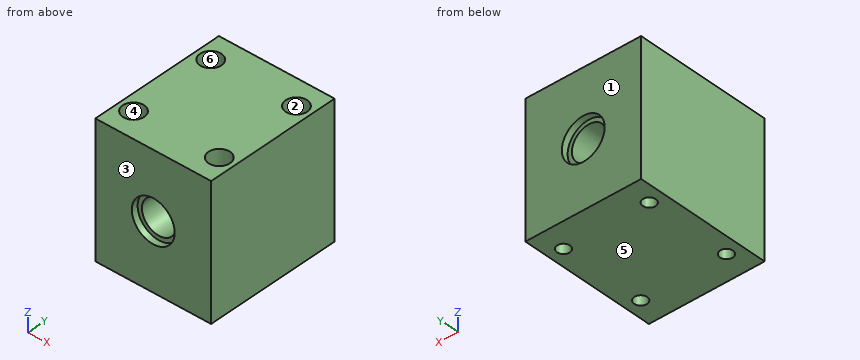
from build123d import *

# Parameters (mm, degrees)
SCHIZZO1_W                   = 27
SCHIZZO1_H                   = 32
ESTRUSIONE_ESTRUSIONE1_DEPTH = 31
SCHIZZO2_R                   = 1.5
TAGLIO_ESTRUSIONE1_DEPTH     = 32
SCHIZZO3_R                   = 4
TAGLIO_ESTRUSIONE2_DEPTH     = 33
SCHIZZO4_R                   = 5
TAGLIO_ESTRUSIONE5_DEPTH     = 1.5
SCHIZZO5_R                   = 5
TAGLIO_ESTRUSIONE6_DEPTH     = 1.5
SCHIZZO6_R                   = 2.5
TAGLIO_ESTRUSIONE7_DEPTH     = 15


with BuildPart() as part:
    # Schizzo1 → Estrusione-Estrusione1 (new body)
    with BuildSketch(Plane.XY):
        Rectangle(SCHIZZO1_W, SCHIZZO1_H)
    extrude(amount=ESTRUSIONE_ESTRUSIONE1_DEPTH)

    # Schizzo2 → Taglio-Estrusione1 (cut, through all)
    with BuildSketch(Plane(origin=(0, 0, 0), x_dir=(-1, 0, 0), z_dir=(0, 0, -1))):
        with Locations((-10, 10)):
            Circle(SCHIZZO2_R)
        with Locations((10, 10)):
            Circle(SCHIZZO2_R)
        with Locations((10, -10)):
            Circle(SCHIZZO2_R)
        with Locations((-10, -10)):
            Circle(SCHIZZO2_R)
    extrude(amount=-TAGLIO_ESTRUSIONE1_DEPTH, mode=Mode.SUBTRACT)

    # Schizzo3 → Taglio-Estrusione2 (cut, through all)
    with BuildSketch(Plane(origin=(0, 16, 0), x_dir=(1, 0, 0), z_dir=(0, 1, 0))):
        with Locations((0, -15.5)):
            Circle(SCHIZZO3_R)
    extrude(amount=-TAGLIO_ESTRUSIONE2_DEPTH, mode=Mode.SUBTRACT)

    # Schizzo4 → Taglio-Estrusione5 (cut)
    with BuildSketch(Plane(origin=(0, 16, 0), x_dir=(1, 0, 0), z_dir=(0, 1, 0))):
        with Locations((0, -15.5)):
            Circle(SCHIZZO4_R)
    extrude(amount=-TAGLIO_ESTRUSIONE5_DEPTH, mode=Mode.SUBTRACT)

    # Schizzo5 → Taglio-Estrusione6 (cut)
    with BuildSketch(Plane.XZ.offset(16)):
        with Locations((0, 15.5)):
            Circle(SCHIZZO5_R)
    extrude(amount=-TAGLIO_ESTRUSIONE6_DEPTH, mode=Mode.SUBTRACT)

    # Schizzo6 → Taglio-Estrusione7 (cut)
    with BuildSketch(Plane.XY.offset(31)):
        with Locations((-10, 10)):
            Circle(SCHIZZO6_R)
        with Locations((10, 10)):
            Circle(SCHIZZO6_R)
        with Locations((10, -10)):
            Circle(SCHIZZO6_R)
        with Locations((-10, -10)):
            Circle(SCHIZZO6_R)
    extrude(amount=-TAGLIO_ESTRUSIONE7_DEPTH, mode=Mode.SUBTRACT)


solid = part.part
Build history of the part. All positions in model axes, mm. Face numbers are marked on the shaded views. A direction names the side the tool comes from. Give positions to 0.01 mm unless a question says otherwise; leave off trailing zeros. Order: outer loops, then holes, each group sorted by start corner. A loop starts at its lowest first (then second) coordinate and runs counter-clockwise, first axis right, second up. Notation, with made-up numbers: M 18,15.25 L 55,15.25 A36 ccw 55,52.25 Z; hole C 50.5,49 d11. An arc over 180 degrees is marked long. Put each result on its own line as item: value.
Item 1: Slice it at B-B, the plane y = 10. Write the cut outline in (x, z).
From the geometry:
outline: M -13.5,0 L -11.5,0 L -11.5,16 L -12.5,16 L -12.5,31 L -13.5,31 Z; M -8.5,0 L 8.5,0 L 8.5,16 L 7.5,16 L 7.5,31 L -7.5,31 L -7.5,16 L -8.5,16 Z; M 11.5,0 L 13.5,0 L 13.5,31 L 12.5,31 L 12.5,16 L 11.5,16 Z; hole C 0,15.5 d8
Item 2: Slice it at D-D, the plane z = 27.5. Write the cut outline in (x, y), plus the area to 3 significant figures.
From the geometry:
outline: M -13.5,-16 L 13.5,-16 L 13.5,16 L -13.5,16 Z; hole C -10,-10 d5; hole C -10,10 d5; hole C 10,-10 d5; hole C 10,10 d5
area: 785 mm2
Item 3: Probe line 1 (Y direction, x = -10, z = 8); line 2 (Y direction, x = -10, z = 23.75); line 3 (X direction, y = -7.5, z = 15.5). List the from-to ranges inside material, lowest first. Write a range as [from, to].
From the geometry:
line 1: y = [-16, -11.5], [-8.5, 8.5], [11.5, 16]
line 2: y = [-16, -12.5], [-7.5, 7.5], [12.5, 16]
line 3: x = [-13.5, -4], [4, 13.5]
Item 4: Flat gauge pins, fed straight in: pin 1 Ø1.5 at (x, y) = (-9.5, -10.5) entering from +Z; pin 2 Ø1.5 at (x, y) = (10, 9) entering from +Z; pin 3 Ø4.5 at (x, y) = (-10, -10) entering from -Z; pin 4 Ø5 at (x, z) = (2, 15.5) entering from -Y. Where does each tip first touch, or does it go through?
From the geometry:
pin 1: passes through
pin 2: stops at z = 16
pin 3: stops at z = 0
pin 4: stops at y = -14.5
Item 5: 3-axis set-ups, long thin cutter, end or side, ignore diameter. For the marked faces 5 and 6: which of +Z, -Z, +X, -X, +Y, -Y reach the whole face in a straight line?
From the geometry:
face 5: -Z, +X, -X, +Y, -Y
face 6: +Z
Item 6: Two-plate mould, pull along Y, no slides. Class the marked faces 1, 2, 3 and 4: +Y half, -Y half, draft (parallel to the pull), parting line (faces both ways), or undercut.
From the geometry:
face 1: +Y half
face 2: undercut
face 3: -Y half
face 4: undercut
Item 7: Slice it at A-A, the plane z = 15.5. Write the cut outline in (x, y), plus the area to 3 significant figures.
From the geometry:
outline: M -13.5,-16 L -5,-16 L -5,-14.5 L -4,-14.5 L -4,14.5 L -5,14.5 L -5,16 L -13.5,16 Z; M 4,-14.5 L 5,-14.5 L 5,-16 L 13.5,-16 L 13.5,16 L 5,16 L 5,14.5 L 4,14.5 Z; hole C -10,-10 d3; hole C -10,10 d3; hole C 10,-10 d3; hole C 10,10 d3
area: 574 mm2
Item 8: Slice it at C-C, the plane x = -10. Write the cut outline in (y, z).
From the geometry:
outline: M -16,0 L -11.5,0 L -11.5,16 L -12.5,16 L -12.5,31 L -16,31 Z; M -8.5,0 L 8.5,0 L 8.5,16 L 7.5,16 L 7.5,31 L -7.5,31 L -7.5,16 L -8.5,16 Z; M 11.5,0 L 16,0 L 16,31 L 12.5,31 L 12.5,16 L 11.5,16 Z
